from build123d import *

# Parameters (mm, degrees)
SKETCH1_R           = 6.35
BOSS_EXTRUDE1_DEPTH = 70
SKETCH2_R           = 15
BOSS_EXTRUDE2_DEPTH = 2.5
BOSS_EXTRUDE3_START = 2.5
SKETCH3_R           = 15
BOSS_EXTRUDE3_DEPTH = 2.5
FILLET1_R           = 8.5


with BuildPart() as part:
    # Sketch1 → Boss-Extrude1 (new body)
    with BuildSketch(Plane.XY):
        Circle(SKETCH1_R)
    extrude(amount=BOSS_EXTRUDE1_DEPTH)

    # Sketch2 → Boss-Extrude2 (add)
    with BuildSketch(Plane(origin=(0, 0, 0), x_dir=(-1, 0, 0), z_dir=(0, 0, -1))):
        Circle(SKETCH2_R)
    extrude(amount=BOSS_EXTRUDE2_DEPTH)

    # Sketch3 → Boss-Extrude3 (add)
    with BuildSketch(Plane.XY.offset(70).offset(BOSS_EXTRUDE3_START)):
        with Locations(Location((0, 0, 0), (0, 0, 180))):
            Circle(SKETCH3_R)
    extrude(amount=-BOSS_EXTRUDE3_DEPTH)

    # Fillet1
    # the kernel refuses this fillet: 8.5 mm, written as the material it takes off along each edge
    with BuildSketch(Plane(origin=(0, 0, 72.5), x_dir=(-1, 0, 0), z_dir=(0, 1, 0))) as fillet1_piece_1:
        with BuildLine():
            CenterArc((8.979202711, -8.5), FILLET1_R, 44.900872156, 45.099127844)
            Line((8.979202711, 0), (8.979202711, 0.17))
            Line((8.979202711, 0.17), (15, 0.17))
            Line((15, 0.17), (15.17, 0))
            ThreePointArc((15.17, 0), (15.17, -1.25), (15.120415946, -2.38))
            Line((15.120415946, -2.38), (15, -2.5))
        make_face()
    revolve(axis=Axis((0, 0, 72.5), (0, 0, 1)), mode=Mode.SUBTRACT)
    with BuildSketch(Plane(origin=(0, 0, -2.5), x_dir=(-1, 0, 0), z_dir=(0, -1, 0))) as fillet1_piece_2:
        with BuildLine():
            CenterArc((8.979202711, -8.5), FILLET1_R, 44.900872156, 45.099127844)
            Line((8.979202711, 0), (8.979202711, 0.17))
            Line((8.979202711, 0.17), (15, 0.17))
            Line((15, 0.17), (15.17, 0))
            ThreePointArc((15.17, 0), (15.17, -1.25), (15.120415946, -2.38))
            Line((15.120415946, -2.38), (15, -2.5))
        make_face()
    revolve(axis=Axis((0, 0, -2.5), (0, 0, -1)), mode=Mode.SUBTRACT)


solid = part.part
Geometry check sheet. Reference: the model listing, model coordinates, mm. Round coordinates to 2 decimals unless told otherwise and drop trailing zeros. Loops run counter-clockwise (first coordinate to the right, second up) from the corner with the lowest first, then second, coordinate; pieces in that order, holes last. Notation, with made-up numbers: (-20.75, 55.5) - (-1.75, 55.5) arc R12 cw to (-1.75, 64.5) - close; hole circle Ø5 at (53.25, 33.25). An arc over 180 degrees is marked (long way). One line per question, with ' | ' between items. Start each with the question number.
1. Cross-section at C-C on z = 9.5. Record the cut outline in (x, y).
2. Cross-section at A-A on y = 0. Record the cut outline in (x, z), then the cut area to 3 significant figures.
3. Draft check along Z on faces 1 (the face through (0, 0, 72.5)), 2 (the face through (-1.38, -6.2, 34.51)), 3 (the face through (0, 0, -2.5)). Enter one of: released by +Z, released by -Z, zero draft, split by the parting line, or undercut.
4. Scan lines: line 1 (Z direction, x = -3, y = 5.75); line 2 (Z direction, x = 12, y = -4.5); line 3 (X direction, y = -0.5, z = 4.5). Record each from-to range of solid material in increasing order. Write a range as [from, to].
5. Depth check by flat-ended pin: pin 1 (10 mm diameter, centred on y = 7.5, z = 56, fed in from -X); pin 2 (10 mm diameter, centred on y = 8.5, z = 19.5, fed in from -X); pin 3 (3 mm diameter, centred on x = 3.5, z = 6.5, fed in from +Y). Enter the tip coordinate at first touch or a pass-through.
Taken from the geometry:
1) outline: circle Ø12.7 at (0, 0)
2) outline: (-15, 0) arc R8.5 ccw to (-8.98, -2.5) - (8.98, -2.5) arc R8.5 ccw to (15, 0) - (6.35, 0) - (6.35, 70) - (15, 70) arc R8.5 ccw to (8.98, 72.5) - (-8.98, 72.5) arc R8.5 ccw to (-15, 70) - (-6.35, 70) - (-6.35, 0) - close | area: 1,020 mm²
3) face 1: released by +Z | face 2: undercut | face 3: released by -Z
4) line 1: [-2.5, 0], [70, 72.5] | line 2: [-1.58, 0], [70, 71.58] | line 3: [-6.33, 6.33]
5) pin 1: x = -5.84 | pin 2: x = -5.3 | pin 3: y = 6.03
